Check sheet for the modelled part. Datum: model origin and axes. Units: mm. Face numbers are marked on the shaded views. A direction names the side the tool comes from. Round coordinates to 2 decimals unless told otherwise and drop trailing zeros. Loops run counter-clockwise (first coordinate to the right, second up) from the corner with the lowest first, then second, coordinate; pieces in that order, holes last. Notation, with made-up numbers: M 57.25,16.5 L 76.25,16.5 A23 ccw 76.25,27.5 Z; hole C -30.75,51.5 d8. An arc over 180 degrees is marked long. One line per question, with ' | ' between items. Start each with the question number.
(1) Thickness scan on probe 1 along Y at (x, z) = (26.5, -31); probe 2 along Z at (x, y) = (47, -33.5); probe 3 along X at (y, z) = (-21, -44.75). Record the ranges inside material, lowest first. Write a range as [from, to].
(2) Draft check along X on the marked faces 1, 2 and 3. Enter one of: +X half, -X half, draft (parallel to the pull), parting line (faces both ways), or undercut.
(3) Go/stop test with flat-tipped pins: P1, Ø8.5, axis at x = -17.5, z = -36.5, coming from the -Y side; P2, Ø5.5, axis at x = -33.74, z = -39.26, coming from the +Y side; P3, Ø3, axis at x = -32, y = -9, coming from the +Z side. Record where each tip stops, or that it passes through.
(4) Section check B-B (x = -11.5). Record the boundary of the cut face in (y, z).
(5) Tool access check on the marked faces 4 and 5. Record the directions out of +Z, -Z, +X, -X, +Y, -Y that give a thin tool (end or side, any length) a straight path to the whole face; none if there is none.
(6) Section check C-C (z = -32.25). Count the separate pieces of the cut face and the enclosed holes in it, and give its area (3 significant figures).
(7) Section check A-A (y = -38). Record the boundary of the cut face in (x, z), and give its area (3 significant figures).
```python
from build123d import *

# Parameters (mm, degrees)
BOSS_EXTRUDE1_DEPTH = 4
SKETCH3_W           = 144
SKETCH3_H           = 5
BOSS_EXTRUDE2_DEPTH = 44.5
SKETCH5_R           = 1.7
CUT_EXTRUDE1_DEPTH  = 4
BOSS_EXTRUDE3_DEPTH = 44.5
FILLET1_R           = 2
FILLET2_R           = 6
FILLET3_R           = 0.5


with BuildPart() as part:
    # Sketch2 → Boss-Extrude1 (new body)
    with BuildSketch(Plane(origin=(0, 0, 0), x_dir=(1, 0, 0), z_dir=(0, 1, 0))):
        with BuildLine():
            Line((72, 30), (72, 54))
            Line((72, 54), (-72, 54))
            Line((-72, 54), (-72, 30))
            Line((-72, 30), (-69.899748742, 30))
            ThreePointArc((-69.899748742, 30), (-50, 36), (-30.100251258, 30))
            Line((-30.100251258, 30), (30.100251258, 30))
            ThreePointArc((30.100251258, 30), (50, 36), (69.899748742, 30))
            Line((69.899748742, 30), (72, 30))
        make_face()
    extrude(amount=BOSS_EXTRUDE1_DEPTH)

    # Sketch3 → Boss-Extrude2 (add)
    with BuildSketch(Plane.XZ):
        with Locations((0, -51.5)):
            Rectangle(SKETCH3_W, SKETCH3_H)
    extrude(amount=BOSS_EXTRUDE2_DEPTH)

    # Sketch5 → Cut-Extrude1 (cut)
    with BuildSketch(Plane(origin=(0, 4, 0), x_dir=(1, 0, 0), z_dir=(0, 1, 0))):
        with Locations(Location((-66.264045876, 39.264880132, 0), (0, 0, 270))):
            Circle(SKETCH5_R)
        with Locations(Location((-33.735954124, 39.264880132, 0), (0, 0, 270))):
            Circle(SKETCH5_R)
        with Locations(Location((33.735954124, 39.264880132, 0), (0, 0, 270))):
            Circle(SKETCH5_R)
        with Locations(Location((66.264045876, 39.264880132, 0), (0, 0, 270))):
            Circle(SKETCH5_R)
    extrude(amount=-CUT_EXTRUDE1_DEPTH, mode=Mode.SUBTRACT)

    # Sketch6 → Boss-Extrude3 (add)
    with BuildSketch(Plane.XZ.offset(44.5)):
        with BuildLine():
            Line((72, -49), (72, -43.783558558))
            ThreePointArc((72, -43.783558558), (61.304990727, -47.678057686), (50, -49))
            Line((50, -49), (72, -49))
        make_face()
        with BuildLine():
            Line((-72, -49), (-50, -49))
            ThreePointArc((-50, -49), (-61.304990727, -47.678057686), (-72, -43.783558558))
            Line((-72, -43.783558558), (-72, -49))
        make_face()
    extrude(amount=-BOSS_EXTRUDE3_DEPTH)

    # Fillet1
    fillet1_edges = [part.edges().sort_by_distance(p)[0] for p in [
        (0, 4, -54),
        (0, 0, -49),
        (61.304990727, 0, -47.678057686),
        (-61.304990727, 0, -47.678057686),
    ]]
    fillet(fillet1_edges, radius=FILLET1_R)

    # Fillet2
    # the kernel refuses this fillet: 6 mm, written as the material it takes off along each edge
    with BuildSketch(Plane(origin=(-72, -11.399550361, -30), x_dir=(0, 0, -1), z_dir=(0, 1, 0))) as fillet2_piece_1:
        with BuildLine():
            CenterArc((4.559820144, -6), FILLET2_R, 90, 49.461555346)
            Line((0, -2.100251258), (-0.091196403, -2.022256283))
            ThreePointArc((-0.091196403, -2.022256283), (-0.12, -1.050125629), (-0.12, 0))
            Line((-0.12, 0), (0, 0.12))
            Line((0, 0.12), (4.559820144, 0.12))
            Line((4.559820144, 0.12), (4.559820144, 0))
        make_face()
    extrude(amount=26.799100721, mode=Mode.SUBTRACT)
    with BuildSketch(Plane(origin=(72, -11.399550361, -30), x_dir=(0, 0, -1), z_dir=(0, 1, 0))) as fillet2_piece_2:
        with BuildLine():
            CenterArc((4.559820144, 6), FILLET2_R, 220.538444654, 49.461555346)
            Line((0, 2.100251258), (-0.091196403, 2.022256283))
            ThreePointArc((-0.091196403, 2.022256283), (-0.12, 1.050125629), (-0.12, 0))
            Line((-0.12, 0), (0, -0.12))
            Line((0, -0.12), (4.559820144, -0.12))
            Line((4.559820144, -0.12), (4.559820144, 0))
        make_face()
    extrude(amount=26.799100721, mode=Mode.SUBTRACT)

    # Fillet3
    fillet3_edges = [part.edges().sort_by_distance(p)[0] for p in [
        (-50, 0, -36),
        (-50, 4, -36),
        (0, 4, -30),
        (50, 4, -36),
        (72, -44.5, -48.891779279),
        (-72, -44.5, -48.891779279),
        (0, -44.5, -54),
        (0, -44.5, -49),
        (61.304990727, -44.5, -47.678057686),
        (-61.304990727, -44.5, -47.678057686),
        (-72, 0, -38.046469729),
        (72, -23.25, -43.783558558),
        (-72, -23.25, -43.783558558),
        (-72, 4, -43.279910072),
        (-72, -21.25, -54),
        (-72, 3.414213562, -53.414213562),
        (72, -21.25, -54),
        (72, 3.414213562, -53.414213562),
        (72, -0.543612491, -43.078170154),
        (-72, -0.543612491, -43.078170154),
        (50, 0, -36),
        (72, 0, -38.046469729),
        (71.44970148, 0, -32.049689914),
        (-71.44970148, 0, -32.049689914),
        (0, 0, -30),
        (72, 4, -43.279910072),
        (71.44970148, 4, -32.049689914),
        (-71.44970148, 4, -32.049689914),
    ]]
    fillet(fillet3_edges, radius=FILLET3_R)


solid = part.part
```
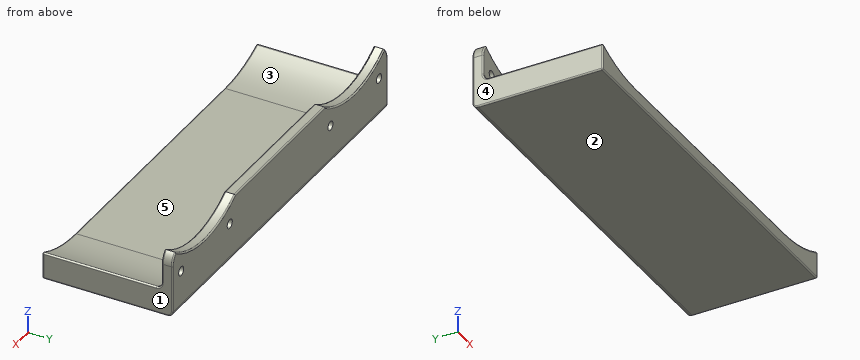
The answers:
1) probe 1: [0, 4] | probe 2: [-54, -49] | probe 3: [-72, -69.96], [69.96, 72]
2) face 1: +X half | face 2: draft | face 3: undercut
3) P1: y = 0 | P2: y = 4 | P3: z = -49
4) outline: M -44.5,-53.5 A0.5 ccw -44,-54 L 2,-54 A2 ccw 4,-52 L 4,-30.5 A0.5 ccw 3.5,-30 L 0.5,-30 A0.5 ccw 0,-30.5 L 0,-47 A2 cw -2,-49 L -44,-49 A0.5 ccw -44.5,-49.5 Z
5) face 4: +Z, -Z, -X, +Y, -Y | face 5: +Z, -Y
6) separate pieces: 3 | enclosed holes: 0 | area: 315 mm²
7) outline: M -72,-53.5 A0.5 ccw -71.5,-54 L 71.5,-54 A0.5 ccw 72,-53.5 L 72,-44.59 A0.5 ccw 71.28,-44.14 A49 cw 50,-49 L -50,-49 A49 cw -71.28,-44.14 A0.5 ccw -72,-44.59 Z | area: 794 mm²
